from build123d import *

# Parameters (mm, degrees)
SKETCH1_W           = 220
SKETCH1_H           = 180
BOSS_EXTRUDE1_DEPTH = 45
FILLET1_R           = 5
SHELL1_T            = -3
CUT_EXTRUDE2_DEPTH  = 5
CUT_EXTRUDE3_DEPTH  = 5
SKETCH4_W           = 11.5
SKETCH4_H           = 6.5
CUT_EXTRUDE4_DEPTH  = 5
SKETCH5_W           = 45.536818034
SKETCH5_H           = 10
CUT_EXTRUDE5_DEPTH  = 5
SKETCH6_W           = 16
SKETCH6_H           = 8.2
CUT_EXTRUDE6_DEPTH  = 5


with BuildPart() as part:
    # Sketch1 → Boss-Extrude1 (new body)
    with BuildSketch(Plane(origin=(0, 0, 0), x_dir=(1, 0, 0), z_dir=(0, 1, 0))):
        with Locations((110, 90)):
            Rectangle(SKETCH1_W, SKETCH1_H)
    extrude(amount=BOSS_EXTRUDE1_DEPTH)

    # Fillet1
    fillet1_edges = [part.edges().sort_by_distance(p)[0] for p in [
        (0, 22.5, -180),
        (220, 22.5, -180),
        (220, 22.5, 0),
        (0, 22.5, 0),
    ]]
    fillet(fillet1_edges, radius=FILLET1_R)

    # Shell1
    shell1_openings = [part.faces().sort_by_distance(p)[0] for p in [
        (110, 45, -90),
    ]]
    offset(amount=SHELL1_T, openings=shell1_openings, kind=Kind.INTERSECTION)

    # Sketch2 → Cut-Extrude2 (cut)
    with BuildSketch(Plane.XY):
        Polygon((175.9, 35), (178.4, 35), (180, 33.4), (180, 24.5), (174.3, 24.5), (174.3, 33.4), align=None)
        Polygon((190.9, 35), (193.4, 35), (195, 33.4), (195, 24.5), (189.3, 24.5), (189.3, 33.4), align=None)
        Polygon((160.9, 35), (163.4, 35), (165, 33.4), (165, 24.5), (159.3, 24.5), (159.3, 33.4), align=None)
        Polygon((145.9, 35), (148.4, 35), (150, 33.4), (150, 24.5), (144.3, 24.5), (144.3, 33.4), align=None)
        Polygon((130.9, 35), (133.4, 35), (135, 33.4), (135, 24.5), (129.3, 24.5), (129.3, 33.4), align=None)
        Polygon((115.9, 35), (118.4, 35), (120, 33.4), (120, 24.5), (114.3, 24.5), (114.3, 33.4), align=None)
        Polygon((100.9, 35), (103.4, 35), (105, 33.4), (105, 24.5), (99.3, 24.5), (99.3, 33.4), align=None)
        Polygon((85.9, 35), (88.4, 35), (90, 33.4), (90, 24.5), (84.3, 24.5), (84.3, 33.4), align=None)
    extrude(amount=-CUT_EXTRUDE2_DEPTH, mode=Mode.SUBTRACT)

    # Sketch3 → Cut-Extrude3 (cut)
    with BuildSketch(Plane.XY):
        Polygon((22.5, 32.9), (36, 32.9), (36, 24.5), (22.5, 24.5), (20, 27), (20, 30.4), align=None)
    extrude(amount=-CUT_EXTRUDE3_DEPTH, mode=Mode.SUBTRACT)

    # Sketch4 → Cut-Extrude4 (cut)
    with BuildSketch(Plane.XY):
        with Locations((51.75, 28.75)):
            Rectangle(SKETCH4_W, SKETCH4_H)
        with Locations((68.55, 28.75)):
            Rectangle(SKETCH4_W, SKETCH4_H)
    extrude(amount=-CUT_EXTRUDE4_DEPTH, mode=Mode.SUBTRACT)

    # Sketch5 → Cut-Extrude5 (cut)
    with BuildSketch(Plane(origin=(220, 0, 0), x_dir=(0, 0, -1), z_dir=(1, 0, 0))):
        with Locations((90, 19.480228536)):
            Rectangle(SKETCH5_W, SKETCH5_H)
    extrude(amount=-CUT_EXTRUDE5_DEPTH, mode=Mode.SUBTRACT)

    # Sketch6 → Cut-Extrude6 (cut)
    with BuildSketch(Plane(origin=(0, 0, -180), x_dir=(-1, 0, 0), z_dir=(0, 0, -1))):
        with Locations((-192, 19.1)):
            Rectangle(SKETCH6_W, SKETCH6_H)
        with Locations((-168, 19.1)):
            Rectangle(SKETCH6_W, SKETCH6_H)
        with Locations((-144, 19.1)):
            Rectangle(SKETCH6_W, SKETCH6_H)
        with Locations((-120, 19.1)):
            Rectangle(SKETCH6_W, SKETCH6_H)
    extrude(amount=-CUT_EXTRUDE6_DEPTH, mode=Mode.SUBTRACT)


solid = part.part
Check sheet for the modelled part. Datum: model origin and axes. Units: mm. A direction names the side the tool comes from. Round coordinates to 2 decimals unless told otherwise and drop trailing zeros. Loops run counter-clockwise (first coordinate to the right, second up) from the corner with the lowest first, then second, coordinate; pieces in that order, holes last. Notation, with made-up numbers: (28.5, 71.5) - (54.5, 71.5) arc R19 ccw to (54.5, 88.5) - close; hole circle Ø11 at (43.25, 76). An arc over 180 degrees is marked (long way). Answer as CSV lines item,"result". Start each with the question number.
Item 1: Release check for a two-part mould opening along Z. For faces 3 (the cylindrical face through (1, 23, -178)), 4 (the cylindrical face through (1, 23, -2)), 5 (the flat face through (217, 28, -89)), 6 (the flat face through (108, 0, -91)) record: +Z half, -Z half, draft (parallel to the pull), parting line (faces both ways), or undercut.
Item 2: Set-up check for faces 1 (the flat face through (109, 22, 0)), 2 (the flat face through (109, 24, -3)): record each of +Z, -Z, +X, -X, +Y, -Y from which the full face is reachable in a straight line by a thin tool's end or side.
Item 3: Section check C-C (y = 37.5). Record the boundary of the cut face in (x, z).
Item 4: Scan lines: line 1 (Z direction, x = 202.5, y = 10.5); line 2 (X direction, y = 32, z = -71.5); line 3 (Y direction, x = 169.5, z = -10). Record each from-to range of solid material in increasing order. Write a range as [from, to].
Item 5: Depth check by flat-ended pin: P1, Ø10, axis at x = 183.5, z = -134, coming from the +Y side; P2, Ø1.5, axis at y = 29.5, z = -2, coming from the -X side; P3, Ø0.9, axis at y = 17.5, z = -178.5, coming from the +X side. Enter the tip coordinate at first touch or a pass-through.
Item 6: Section check B-B (z = -83). Record the boundary of the cut face in (x, y).
Item 7: Section check D-D (x = 42). Record the boundary of the cut face in (y, z).
Item 8: Section check A-A (x = 139). Record the boundary of the cut face in (y, z).
Report:
1,face 3,"-Z half"
1,face 4,"+Z half"
1,face 5,"undercut"
1,face 6,"draft"
2,face 1,"+Z, +X, -X, +Y, -Y"
2,face 2,"+Y"
3,outline,"(0, -175) arc R5 ccw to (5, -180) - (215, -180) arc R5 ccw to (220, -175) - (220, -5) arc R5 ccw to (215, 0) - (5, 0) arc R5 ccw to (0, -5) - close; hole (3, -175) arc R2 ccw to (5, -177) - (215, -177) arc R2 ccw to (217, -175) - (217, -5) arc R2 ccw to (215, -3) - (5, -3) arc R2 ccw to (3, -5) - close"
4,line 1,"z = [-180, -177], [-3, 0]"
4,line 2,"x = [0, 3], [217, 220]"
4,line 3,"y = [0, 3]"
5,P1,"stops at y = 3"
5,P2,"stops at x = 0.53"
5,P3,"stops at x = 218.96"
6,outline,"(0, 0) - (220, 0) - (220, 14.48) - (217, 14.48) - (217, 3) - (3, 3) - (3, 45) - (0, 45) - close; (217, 24.48) - (220, 24.48) - (220, 45) - (217, 45) - close"
7,outline,"(0, -180) - (45, -180) - (45, -177) - (3, -177) - (3, -3) - (45, -3) - (45, 0) - (0, 0) - close"
8,outline,"(0, -180) - (15, -180) - (15, -177) - (3, -177) - (3, -3) - (45, -3) - (45, 0) - (0, 0) - close; (23.2, -180) - (45, -180) - (45, -177) - (23.2, -177) - close"
